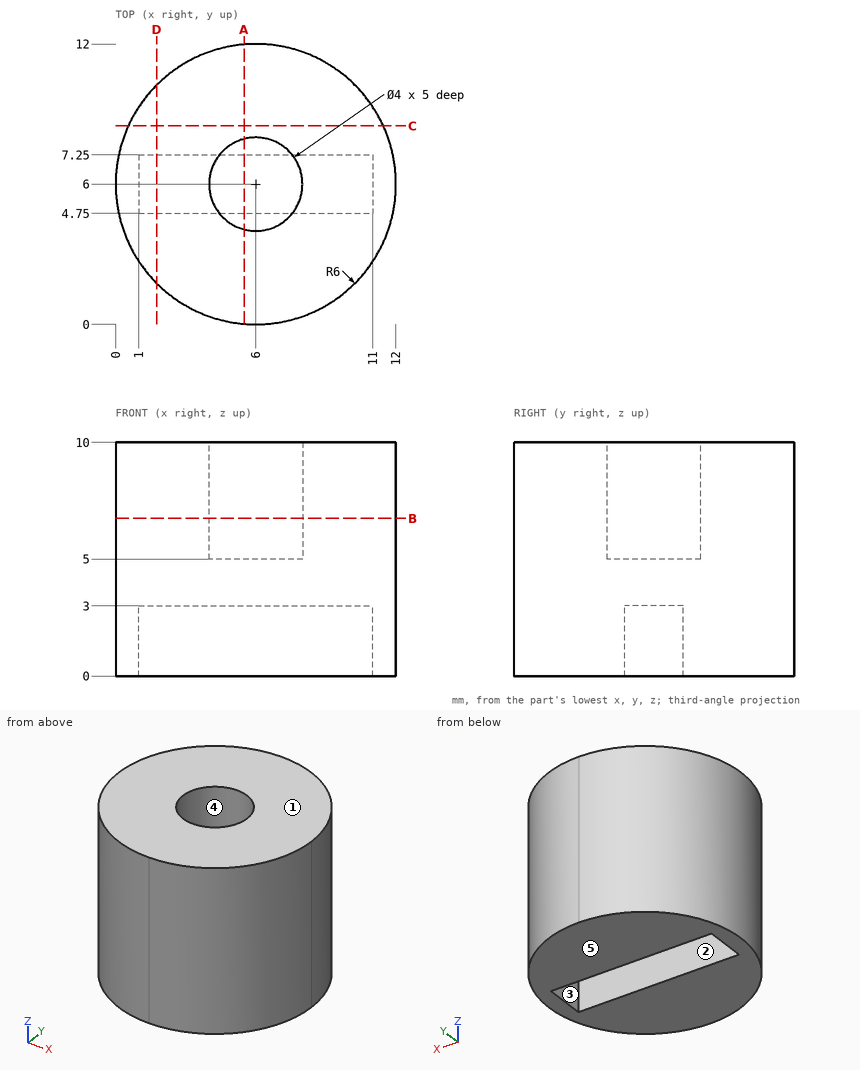
The drawing under review shows one solid part. Ordinate dimensions are in mm from its lowest x, y, z. A direction names the side the tool comes from. Round coordinates to 2 decimals unless told otherwise and drop trailing zeros. Write each loop counter-clockwise with the first axis right and the second up, starting at its lowest first coordinate (ties: lowest second). Pieces come first, ordered by that corner, then holes. Notation, with made-up numbers: (-37.5, 52) - (10.5, 52) arc R28 ccw to (10.5, 70) - close; hole circle Ø5 at (80.25, 42). An arc over 180 degrees is marked (long way). Use one line per item in the form item = value.
Q1. Draft analysis for pull direction X (two halves, no side actions). For the marked faces 1, 2 and 3, state which applies: +X half, -X half, draft (parallel to the pull), parting line (faces both ways), or undercut.
Answer key:
face_1 = draft
face_2 = undercut
face_3 = undercut
Q2. For line 1 (Y direction, x = 6, z = 7.4); line 2 (Y direction, x = 1.25, z = 1.25); line 3 (Z direction, x = 3, y = 5.75), list the stretches that pass through material, from the lowest coordinate up. Write a range as [from, to].
Answer key:
line_1 = [0, 4], [8, 12]
line_2 = [2.33, 4.75], [7.25, 9.67]
line_3 = [3, 10]
Q3. Consider section C-C (y = 8.5). State the section outline as (x, z) points.
Answer key:
outline = (0.55, 0) - (11.45, 0) - (11.45, 10) - (0.55, 10) - close
Q4. Consider section B-B (z = 6.75). State the section outline as (x, y) points.
Answer key:
outline = (6, 0) arc R6 ccw to (12, 6) arc R6 ccw to (6, 12) arc R6 ccw to start; hole circle Ø4 at (6, 6)
Q5. Consider section A-A (x = 5.5). State the section outline as (y, z) points.
Answer key:
outline = (0.02, 0) - (4.75, 0) - (4.75, 3) - (7.25, 3) - (7.25, 0) - (11.98, 0) - (11.98, 10) - (7.94, 10) - (7.94, 5) - (4.06, 5) - (4.06, 10) - (0.02, 10) - close
Q6. Tool access review of the marked faces 4 and 5: name each direction out of +Z, -Z, +X, -X, +Y, -Y from which nothing blocks a thin tool from reaching the whole face with its end or side.
Answer key:
face_4 = +Z
face_5 = -Z, +X, -X, +Y, -Y
Q7. Consider section D-D (x = 1.75). State the section outline as (y, z) points.
Answer key:
outline = (1.76, 0) - (4.75, 0) - (4.75, 3) - (7.25, 3) - (7.25, 0) - (10.24, 0) - (10.24, 10) - (1.76, 10) - close
Q8. Insertion check: pin 1 Ø1.5 at (x, z) = (7.5, 2) entering from -Y; pin 2 Ø1.2 at (x, y) = (5.5, 6.5) entering from -Z; pin 3 Ø4 at (y, z) = (8.5, 6.5) entering from +X; pin 4 Ø3 at (x, y) = (6, 6) entering from -Z. Each pin has a flat end and moves straight along its axis. Give the tip position at first contact, or say it passes through.
Answer key:
pin_1 = 0.05
pin_2 = 3
pin_3 = 11.98
pin_4 = 0
